from build123d import *

# Parameters (mm, degrees)
CUT_EXTRUDE1_REACH = 71.527
SKETCH2_R          = 4.5


with BuildPart() as part:
    # Sketch1 → Revolve1 (revolve)
    with BuildSketch(Plane.XY, mode=Mode.PRIVATE) as revolve1_sk:
        Polygon((-45, 28), (-45, 22), (-29.5, 22), (-29.5, 20.5), (-31, 20.5), (-31, 0), (-26.320011027, 0), (-22, 24.5), (0, 24.5), (0, 27), (-27, 27), (-27, 28), align=None)
    revolve(revolve1_sk.sketch.rotate(Axis((0, 30.618797564, 0), (0, -1, 0)), 270), axis=Axis((0, 30.618797564, 0), (0, -1, 0)))

    # Sketch2 → Cut-Extrude1 (cut, up to next)
    with BuildSketch(Plane(origin=(0, 28, 0), x_dir=(1, 0, 0), z_dir=(0, 1, 0)), mode=Mode.PRIVATE) as cut_extrude1_sk1:
        with Locations(Location((0, 37, 0), (0, 0, 270))):
            Circle(SKETCH2_R)
    cut_extrude1_tool1 = extrude(cut_extrude1_sk1.sketch, amount=-CUT_EXTRUDE1_REACH, mode=Mode.PRIVATE) & part.part
    # Sketch2 → Cut-Extrude1 (cut, up to next)
    with BuildSketch(Plane(origin=(0, 28, 0), x_dir=(1, 0, 0), z_dir=(0, 1, 0)), mode=Mode.PRIVATE) as cut_extrude1_sk2:
        with Locations(Location((32.04293994, 18.5, 0), (0, 0, 270))):
            Circle(SKETCH2_R)
    cut_extrude1_tool2 = extrude(cut_extrude1_sk2.sketch, amount=-CUT_EXTRUDE1_REACH, mode=Mode.PRIVATE) & part.part
    # Sketch2 → Cut-Extrude1 (cut, up to next)
    with BuildSketch(Plane(origin=(0, 28, 0), x_dir=(1, 0, 0), z_dir=(0, 1, 0)), mode=Mode.PRIVATE) as cut_extrude1_sk3:
        with Locations(Location((32.04293994, -18.5, 0), (0, 0, 270))):
            Circle(SKETCH2_R)
    cut_extrude1_tool3 = extrude(cut_extrude1_sk3.sketch, amount=-CUT_EXTRUDE1_REACH, mode=Mode.PRIVATE) & part.part
    # Sketch2 → Cut-Extrude1 (cut, up to next)
    with BuildSketch(Plane(origin=(0, 28, 0), x_dir=(1, 0, 0), z_dir=(0, 1, 0)), mode=Mode.PRIVATE) as cut_extrude1_sk4:
        with Locations(Location((0, -37, 0), (0, 0, 270))):
            Circle(SKETCH2_R)
    cut_extrude1_tool4 = extrude(cut_extrude1_sk4.sketch, amount=-CUT_EXTRUDE1_REACH, mode=Mode.PRIVATE) & part.part
    # Sketch2 → Cut-Extrude1 (cut, up to next)
    with BuildSketch(Plane(origin=(0, 28, 0), x_dir=(1, 0, 0), z_dir=(0, 1, 0)), mode=Mode.PRIVATE) as cut_extrude1_sk5:
        with Locations(Location((-32.04293994, -18.5, 0), (0, 0, 270))):
            Circle(SKETCH2_R)
    cut_extrude1_tool5 = extrude(cut_extrude1_sk5.sketch, amount=-CUT_EXTRUDE1_REACH, mode=Mode.PRIVATE) & part.part
    # Sketch2 → Cut-Extrude1 (cut, up to next)
    with BuildSketch(Plane(origin=(0, 28, 0), x_dir=(1, 0, 0), z_dir=(0, 1, 0)), mode=Mode.PRIVATE) as cut_extrude1_sk6:
        with Locations(Location((-32.04293994, 18.5, 0), (0, 0, 270))):
            Circle(SKETCH2_R)
    cut_extrude1_tool6 = extrude(cut_extrude1_sk6.sketch, amount=-CUT_EXTRUDE1_REACH, mode=Mode.PRIVATE) & part.part
    add(cut_extrude1_tool1.solids().sort_by_distance((0, 28, -37))[0], mode=Mode.SUBTRACT)
    add(cut_extrude1_tool2.solids().sort_by_distance((32.04294, 28, -18.5))[0], mode=Mode.SUBTRACT)
    add(cut_extrude1_tool3.solids().sort_by_distance((32.04294, 28, 18.5))[0], mode=Mode.SUBTRACT)
    add(cut_extrude1_tool4.solids().sort_by_distance((0, 28, 37))[0], mode=Mode.SUBTRACT)
    add(cut_extrude1_tool5.solids().sort_by_distance((-32.04294, 28, 18.5))[0], mode=Mode.SUBTRACT)
    add(cut_extrude1_tool6.solids().sort_by_distance((-32.04294, 28, -18.5))[0], mode=Mode.SUBTRACT)


solid = part.part
Could you check a few things on this model? Use its own coordinates, in mm. A direction names the side the tool comes from. Give positions to 0.01 mm unless a question says otherwise; leave off trailing zeros. Order: outer loops, then holes, each group sorted by start corner. A loop starts at its lowest first (then second) coordinate and runs counter-clockwise, first axis right, second up. Notation, with made-up numbers: (56, 20) - (112, 20) arc R19 ccw to (112, 44) - close; hole circle Ø3 at (-38, 26). An arc over 180 degrees is marked (long way). One line per item, written item: value. Start each with the question number.
1. If I drill on probe 1 along Y at (x, z) = (17.5, -24.5); probe 2 along X at (y, z) = (26.15, -18.5); probe 3 along Z at (x, y) = (36, 23.25), over which ranges is the centre line in solid material (lowest first)?
2. Thinking about a two-plate mould opening in Z: for faces 1 (the face through (11.34, 20.5, -27.41)), 2 (the face through (-30.736, 10.106, -4.036)), 3 (the face through (0, 24.5, 0)), 4 (the face through (-34.78, 25.04, -22.07)), which applies, +Z half, -Z half, draft (parallel to the pull), parting line (faces both ways), or undercut?
3. Imagine slicing it at B-B on x = 0. List the corners of the cut face in (y, z) for me.
4. Imagine slicing it at C-C on z = 0. List the corners of the cut face in (x, y) for me.
5. For P1, Ø1, axis at x = -8.5, y = 17.5, coming from the -Z side; P2, Ø5.5, axis at x = -32.04, z = -18.5, coming from the +Y side; P3, Ø8, axis at y = 5, z = 13, coming from the -X side; P4, Ø6, axis at x = -13.5, y = 25, coming from the +Z side, each with a flat end and sliding along its axis, tell me the tip position at first contact or that it passes through.
6. Imagine slicing it at D-D on y = 12. List the corners of the cut face in (x, z) for me, plus the area to 3 significant figures.
7. Imagine slicing it at A-A on z = -38.5. List the corners of the cut face in (x, y) for me.
8. For faces 5 (the face through (26.36, 27.51, -5.85)), 6 (the face through (9, 22, 29)), 7 (the face through (1.352, 25.042, 41.292)), which set-ups out of +Z, -Z, +X, -X, +Y, -Y let a thin tool reach every point of the face, with its end or its side?
Values:
1. probe 1: 0 to 20.5, 22 to 28
1. probe 2: -41.02 to -36.54, -27.54 to 27.54, 36.54 to 41.02
1. probe 3: -27 to -20.64, -16.36 to 16.36, 20.64 to 27
2. face 1: draft
2. face 2: parting line
2. face 3: undercut
2. face 4: undercut
3. outline: (0, -31) - (20.5, -31) - (20.5, -29.5) - (22, -29.5) - (22, -32.5) - (28, -32.5) - (28, -27) - (27, -27) - (27, 27) - (28, 27) - (28, 32.5) - (22, 32.5) - (22, 29.5) - (20.5, 29.5) - (20.5, 31) - (0, 31) - (0, 26.32) - (24.5, 22) - (24.5, -22) - (0, -26.32) - close; (22, -45) - (28, -45) - (28, -41.5) - (22, -41.5) - close; (22, 41.5) - (28, 41.5) - (28, 45) - (22, 45) - close
4. outline: (-45, 22) - (-29.5, 22) - (-29.5, 20.5) - (-31, 20.5) - (-31, 0) - (-26.32, 0) - (-22, 24.5) - (22, 24.5) - (26.32, 0) - (31, 0) - (31, 20.5) - (29.5, 20.5) - (29.5, 22) - (45, 22) - (45, 28) - (27, 28) - (27, 27) - (-27, 27) - (-27, 28) - (-45, 28) - close
5. P1: z = -29.95
5. P2: through
5. P3: x = -29.66
5. P4: z = 43.76
6. outline: circle Ø62 at (0, 0); hole circle Ø48.41 at (0, 0)
6. area: 1,180 mm²
7. outline: (-23.3, 22) - (-4.24, 22) - (-4.24, 28) - (-23.3, 28) - close; (4.24, 22) - (23.3, 22) - (23.3, 28) - (4.24, 28) - close
8. face 5: +Y
8. face 6: none
8. face 7: +Y, -Y
